from build123d import *

# Parameters (mm, degrees)
CYLINDER026_R                      = 1.5
CYLINDER026_DEPTH                  = 19
CYLINDER025_R                      = 2.84
CYLINDER025_DEPTH                  = 3
FUSION001018017023_PLACEMENT_ANGLE = 180
POCKET002018004005005017_DEPTH     = 2


with BuildPart() as cylinder026:
    # Cylinder026 → Cylinder026 (new body)
    with BuildSketch(Plane.XY):
        Circle(CYLINDER026_R)
    extrude(amount=CYLINDER026_DEPTH)


with BuildPart() as zylinderkopfschraube_m3x16_din912:
    # Cylinder025 → Cylinder025 (new body)
    with BuildSketch(Plane.XY):
        Circle(CYLINDER025_R)
    extrude(amount=CYLINDER025_DEPTH)

    # Fusion001018017023: union Cylinder026
    add(cylinder026.part)


with BuildPart() as zylinderkopfschraube_m3x16_din912_1:
    # Fusion001018017023 placement: moved
    add(zylinderkopfschraube_m3x16_din912.part.rotate(Axis((0, 0, 0), (0, 1, 0)), FUSION001018017023_PLACEMENT_ANGLE))

    # Sketch025 → Pocket002018004005005017 (cut)
    with BuildSketch(Plane(origin=(0, 0, 0), x_dir=(-1, 0, 0), z_dir=(0, 0, 1))):
        Polygon((1.25, -0.721688), (1.25, 0.721688), (0, 1.443376), (-1.25, 0.721688), (-1.25, -0.721688), (0, -1.443376), align=None)
    extrude(amount=-POCKET002018004005005017_DEPTH, mode=Mode.SUBTRACT)


solid = zylinderkopfschraube_m3x16_din912_1.part
The model under review builds one solid part; all positions refer to its coordinate system, in mm. A direction names the side the tool comes from. Coordinates: 2 decimals unless noted, no trailing zeros. Write each loop counter-clockwise with the first axis right and the second up, starting at its lowest first coordinate (ties: lowest second). Pieces come first, ordered by that corner, then holes. Notation, with made-up numbers: (78.5, 18) - (109.5, 18) arc R20 ccw to (109.5, 46) - close; hole circle Ø7 at (18, -9.5). An arc over 180 degrees is marked (long way). Answer as a JSON object with one key per item and string values. Group by question number.
1. Add section A-A (z = -1.5). Give the boundary of the cut face in (x, y), plus the area to 3 significant figures.
2. Mouldability with a two-part tool opening along Y and no side actions: class faces 1 (the face through (2.837, 0.125, -1.479)), 2 (the face through (-0.616, 1.088, -0.986)), 3 (the face through (-1.2, -1.2, -3)) as pulls with the +Y half, pulls with the -Y half, needs draft (parallel to the pull), parting line crosses it, or undercut.
3. Machinability: for faces 4 (the face through (-0.6, 1.3, 0)), 5 (the face through (1.2, -0.9, -10.9)), 6 (the face through (-1.25, 0, -1)), which of the approach directions +Z, -Z, +X, -X, +Y, -Y give a long, thin tool a straight path to every point of the face, cutting with its end or side? Answer none if there is none.
4. Clearance check with flat-ended pins moving along their axes: pin 1 Ø1.6 at (y, z) = (0.5, -0.5) entering from +X; pin 2 Ø1.2 at (x, y) = (0.5, 0) entering from +Z; pin 3 Ø2 at (y, z) = (-1.5, -5) entering from +X. State where each tip first meets the part, or that it passes through.
5. To check wall thickness, follow probe 1 along Z at (x, y) = (-0.8, 2.1); probe 2 along X at (y, z) = (0.6, -1.25); probe 3 along X at (y, z) = (-0.4, -11.5). State the ranges of each line that lie inside material, in increasing order.
6. Add section C-C (x = 0.2). Give the boundary of the cut face in (y, z), plus the area to 3 significant figures.
7. Add section B-B (y = 0). Give the boundary of the cut face in (x, z), plus the area to 3 significant figures.
8. Add section D-D (z = -14.5). Give the boundary of the cut face in (x, y), plus the area to 3 significant figures.
Findings:
{
 "1": {"outline": "circle Ø5.68 at (0, 0); hole (-1.25, -0.72) - (0, -1.44) - (1.25, -0.72) - (1.25, 0.72) - (0, 1.44) - (-1.25, 0.72) - close", "area": "19.9 mm²"},
 "2": {"face 1": "parting line crosses it", "face 2": "undercut", "face 3": "needs draft"},
 "3": {"face 4": "+Z, +X, -X, +Y, -Y", "face 5": "-Z", "face 6": "+Z"},
 "4": {"pin 1": "x = 2.84", "pin 2": "z = -2", "pin 3": "x = 1.41"},
 "5": {"probe 1": "-3 to 0", "probe 2": "-2.78 to -1.25, 1.25 to 2.78", "probe 3": "-1.45 to 1.45"},
 "6": {"outline": "(-2.83, -3) - (-1.49, -3) - (-1.49, -19) - (1.49, -19) - (1.49, -3) - (2.83, -3) - (2.83, 0) - (1.33, 0) - (1.33, -2) - (-1.33, -2) - (-1.33, 0) - (-2.83, 0) - close", "area": "59.3 mm²"},
 "7": {"outline": "(-2.84, -3) - (-1.5, -3) - (-1.5, -19) - (1.5, -19) - (1.5, -3) - (2.84, -3) - (2.84, 0) - (1.25, 0) - (1.25, -2) - (-1.25, -2) - (-1.25, 0) - (-2.84, 0) - close", "area": "60.0 mm²"},
 "8": {"outline": "circle Ø3 at (0, 0)", "area": "7.07 mm²"}
}
